Geometry check sheet. Reference: drawing and pictorial views, mm from the part's lowest x, y, z. Give positions to 0.01 mm unless a question says otherwise; leave off trailing zeros. Write each loop counter-clockwise with the first axis right and the second up, starting at its lowest first coordinate (ties: lowest second). Pieces come first, ordered by that corner, then holes. Notation, with made-up numbers: (-25.75, 57.25) -> (24.25, 57.25) arc R29 ccw to (24.25, 79.25) -> close; hole circle Ø5 at (-24, -35). An arc over 180 degrees is marked (long way). Use a Markdown table: item, result. Add a question column.
1. Gauge pin test, flat ends, axial feed: P1, Ø5, axis at y = 21, z = 4.5, coming from the -X side; P2, Ø5, axis at x = 15.5, z = 7, coming from the -Y side; P3, Ø1, axis at x = 15, z = 6.5, coming from the +Y side. Record the tip position at first contact, or that the pin passes through.
2. Cross-section at A-A (y = 26). Enter the section's corners in (x, z).
3. Cross-section at C-C (z = 5.5). Enter the section's corners in (x, y), then the cut area to 3 significant figures.
4. Scan lines: probe 1 along Y at (x, z) = (26, 0.35); probe 2 along Y at (x, z) = (26, 6.45); probe 3 along X at (y, z) = (14.5, 7). Record each from-to range of solid material in increasing order. Write a range as [from, to].
5. Release check for a two-part mould opening along Y. For the marked faces 1, 2 and 3 record: released by +Y, released by -Y, zero draft, split by the parting line, or undercut.
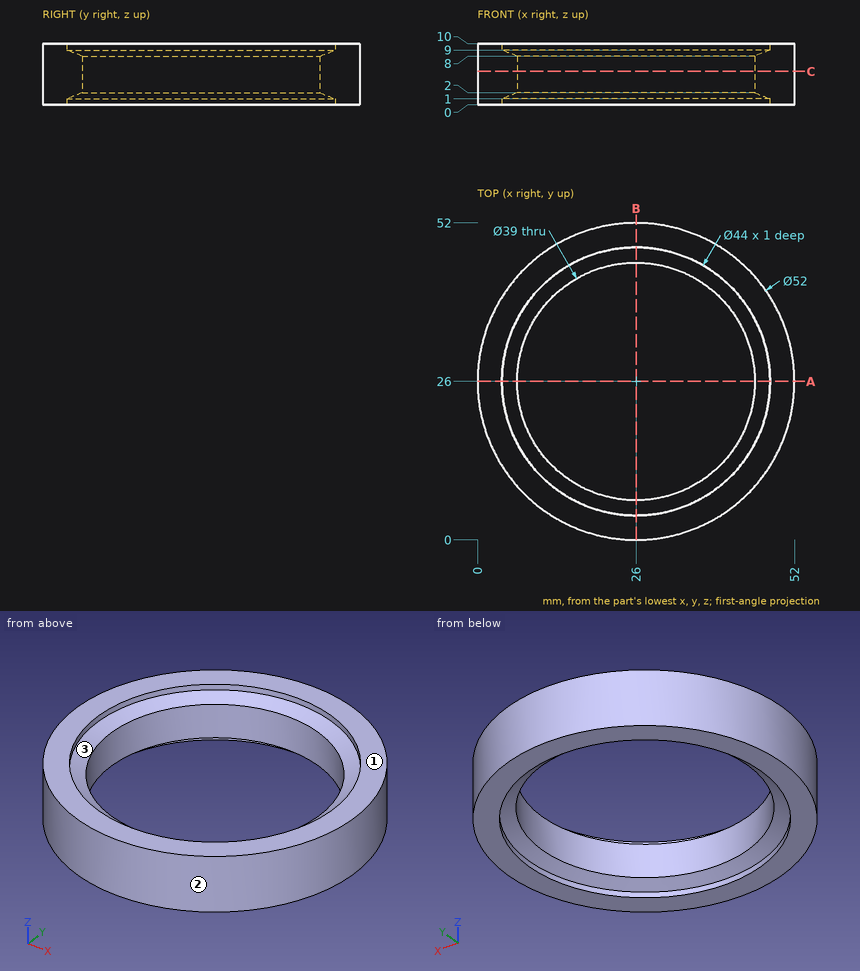
Worked answers:
| question | item | result |
|---|---|---|
| 1 | P1 | stops at x = 0.12 |
| 1 | P2 | stops at y = 1.26 |
| 1 | P3 | stops at y = 49.79 |
| 2 | outline | (0, 0) -> (4, 0) -> (4, 1) -> (6.5, 2) -> (6.5, 8) -> (4, 9) -> (4, 10) -> (0, 10) -> close; (45.5, 2) -> (48, 1) -> (48, 0) -> (52, 0) -> (52, 10) -> (48, 10) -> (48, 9) -> (45.5, 8) -> close |
| 3 | outline | circle Ø52 at (26, 26); hole circle Ø39 at (26, 26) |
| 3 | area | 929 mm² |
| 4 | probe 1 | y = [0, 4], [48, 52] |
| 4 | probe 2 | y = [0, 6.5], [45.5, 52] |
| 4 | probe 3 | x = [2.68, 10.25], [41.75, 49.32] |
| 5 | face 1 | zero draft |
| 5 | face 2 | split by the parting line |
| 5 | face 3 | undercut |
